Can you work these out from the model? Positions are in its coordinate system, mm. A direction names the side the tool comes from. Coordinates: 2 decimals unless noted, no trailing zeros. Order: outer loops, then holes, each group sorted by start corner. A loop starts at its lowest first (then second) coordinate and runs counter-clockwise, first axis right, second up. Notation, with made-up numbers: (-21.75, -19) -> (14.25, -19) arc R17 cw to (14.25, -3) -> close; hole circle Ø9 at (77, 50). An arc over 180 degrees is marked (long way). Write item = value, one per line. Start each with the question number.
from build123d import *

# Parameters (mm, degrees)
F2_DEPTH = 25.4
F3_DEPTH = 25.4


with BuildPart() as f2:
    # F0 (on Front) → F2 (new body, symmetric)
    with BuildSketch(Plane.XZ):
        Polygon((-4.459682, 25.4), (-22.225, -25.4), (-15.367, -25.4), (-8.882659, -6.858), (0, -6.858), (8.882659, -6.858), (15.367, -25.4), (22.225, -25.4), (4.459682, 25.4), (0, 25.4), align=None)
        Polygon((-6.484341, 0), (0, 18.542), (6.484341, 0), (0, 0), align=None, mode=Mode.SUBTRACT)
    extrude(amount=F2_DEPTH, both=True)

    # F1 (on Right) → F3 (intersect, symmetric)
    with BuildSketch(Plane.YZ):
        with BuildLine():
            Line((10.950837, 12.134485), (17.372236, 14.542348))
            ThreePointArc((17.372236, 14.542348), (3.210506, 24.639486), (-11.470547, 15.313531))
            ThreePointArc((-11.470547, 15.313531), (-14.831433, -0.761551), (-11.470547, -16.836634))
            ThreePointArc((-11.470547, -16.836634), (1.458806, -26.099206), (15.7648, -19.149246))
            Line((15.7648, -19.149246), (10.034468, -15.38156))
            ThreePointArc((10.034468, -15.38156), (2.039045, -19.265796), (-5.186992, -14.089072))
            ThreePointArc((-5.186992, -14.089072), (-7.973433, -0.761551), (-5.186992, 12.56597))
            ThreePointArc((-5.186992, 12.56597), (3.027206, 17.783936), (10.950837, 12.134485))
        make_face()
    extrude(amount=F3_DEPTH, both=True, mode=Mode.INTERSECT)


solid = f2.part
(1) Imagine slicing it at B-B (z = -18.5). Write out the boundary of the cut face in (x, y), plus the area to 3 significant figures.
(2) Imagine slicing it at C-C (y = 12). Write out the boundary of the cut face in (x, z).
(3) For P1, Ø6, axis at x = -6.5, y = 0.5, coming from the -Z side; P2, Ø1, axis at x = -1.5, y = 9, coming from the -Z side; P3, Ø7.5, axis at x = 2, y = -12.5, coming from the -Z side, each with a flat end and sliding along its axis, tell me the tip position at first contact or that it passes through.
(4) Thinking about a two-plate mould opening in Y: for faces 1 (the face through (-5.195, 14.117, 13.322)), 2 (the face through (19, 3, -25.4)), 3 (the face through (15.941, 2.169, -19.276)), 4 (the face through (17.37, -7.73, -22.07)), which applies, +Y half, -Y half, draft (parallel to the pull), parting line (faces both ways), or undercut?
(5) For faces 5 (the face through (0, -11, -6.858)), 6 (the face through (-4.453, 2.883, 17.787)), 7 (the face through (0, -11, 0)), which set-ups out of +Z, -Z, +X, -X, +Y, -Y let a thin tool reach every point of the face, with its end or its side?
(6) Imagine slicing it at D-D (z = -7.5). Write out the boundary of the cut face in (x, y), plus the area to 3 significant figures.
(7) If I drill on L1, parallel to X at y = -8.5, z = -13; L2, parallel to X at y = -13, z = -7.5; L3, parallel to Y at x = 7, z = 0, over which ranges is the centre line in solid material (lowest first)? Write a range as from..to.
(8) Imagine slicing it at A-A (x = -5.5). Write out the boundary of the cut face in (y, z).
Result set:
q1.outline = (-19.81, -10.62) -> (-12.95, -10.62) -> (-12.95, -0.86) -> (-19.81, -0.86) -> close; (-19.81, 6.41) -> (-12.95, 6.41) -> (-12.95, 14.78) -> (-19.81, 14.78) -> close; (12.95, -10.62) -> (19.81, -10.62) -> (19.81, -0.86) -> (12.95, -0.86) -> close; (12.95, 6.41) -> (19.81, 6.41) -> (19.81, 14.78) -> (12.95, 14.78) -> close
q1.area = 249 mm2
q2.outline = (-21.43, -23.12) -> (-14.57, -23.12) -> (-12.32, -16.67) -> (-19.17, -16.67) -> close; (-8.96, 12.53) -> (-2.1, 12.53) -> (0, 18.54) -> (2.1, 12.53) -> (8.96, 12.53) -> (5.78, 21.63) -> (-5.78, 21.63) -> close; (12.32, -16.67) -> (14.57, -23.12) -> (21.43, -23.12) -> (19.17, -16.67) -> close
q3.P1 = 15.99
q3.P2 = 14.64
q3.P3 = -6.86
q4.face_1 = +Y half
q4.face_2 = draft
q4.face_3 = undercut
q4.face_4 = -Y half
q5.face_5 = -Z, +Y, -Y
q5.face_6 = -Z, +X, -X
q5.face_7 = +Y, -Y
q6.outline = (-15.97, -14.26) -> (-9.11, -14.26) -> (-9.11, -7.28) -> (-15.97, -7.28) -> close; (9.11, -14.26) -> (15.97, -14.26) -> (15.97, -7.28) -> (9.11, -7.28) -> close
q6.area = 95.7 mm2
q7.L1 = -17.89..-11.03, 11.03..17.89
q7.L2 = -15.97..-9.11, 9.11..15.97
q7.L3 = -14.82..-7.96
q8.outline = (-14.82, 0) arc R40.12 ccw to (-14.37, -6.86) -> (-7.41, -6.86) arc R33.27 cw to (-7.96, 0) -> close; (-14.67, 2.81) -> (-7.78, 2.81) arc R33.27 cw to (-5.19, 12.57) arc R8.71 cw to (10.95, 12.13) -> (17.37, 14.54) arc R15.57 ccw to (10.81, 22.43) -> (-5.22, 22.43) arc R15.57 ccw to (-11.47, 15.31) arc R40.12 ccw to start
